from build123d import *

# Parameters (mm, degrees)
WYTNIJ_WYCI_GNI_CIE1_START = -52
WYTNIJ_WYCI_GNI_CIE1_DEPTH = 72
SZKIC3_R                   = 3
WYTNIJ_WYCI_GNI_CIE2_DEPTH = 12
SZYK_KO_OWY1_COUNT         = 6


with BuildPart() as part:
    # Szkic1 → Obrót1 (revolve)
    with BuildSketch(Plane.XY):
        Polygon((0, -4), (0, -9.4775), (1, -10.4775), (6.5225, -10.4775), (8, -9), (10, -9), (10, -11.1), (10.489897949, -11.5), (10, -12.1), (10, -12.5), (19, -12.5), (19, -15.585), (28.915, -15.585), (32, -12.5), (70, -12.5), (70, -11.3155), (68, -9.3155), (54, -9.3155), (53, -10.5), (50, -10.5), (50, -8.5), (19, -8.5), (19, -8.1), (22, -5), (19, -5), (19, -4), align=None)
    revolve(axis=Axis((0, 0, 0), (1, 0, 0)))

    # Szkic2 → Wytnij-wyciągnięcie1 (cut)
    with BuildSketch(Plane.ZY.offset(-19).offset(WYTNIJ_WYCI_GNI_CIE1_START)):
        Polygon((-92.411763114, 13.5), (-7.787311795, 13.5), (7.787311795, 13.5), (92.411763114, 13.5), (92.411763114, 182.748902638), (-92.411763114, 182.748902638), align=None)
    wytnij_wyci_gni_cie1 = extrude(amount=WYTNIJ_WYCI_GNI_CIE1_DEPTH, mode=Mode.SUBTRACT)

    # Szkic3 → Wytnij-wyciągnięcie2 (cut)
    with BuildSketch(Plane(origin=(0, 13.5, 0), x_dir=(1, 0, 0), z_dir=(0, 1, 0))):
        with Locations((25, 0)):
            Circle(SZKIC3_R)
    wytnij_wyci_gni_cie2 = extrude(amount=-WYTNIJ_WYCI_GNI_CIE2_DEPTH, mode=Mode.SUBTRACT)

    # Szyk kołowy1: Wytnij-wyciągnięcie1, Wytnij-wyciągnięcie2 ×6 about axis
    szyk_ko_owy1_axis = Axis((0, 0, 0), (-1, 0, 0))
    for i in range(1, SZYK_KO_OWY1_COUNT):
        add(wytnij_wyci_gni_cie1.rotate(szyk_ko_owy1_axis, i * 360 / SZYK_KO_OWY1_COUNT), mode=Mode.SUBTRACT)
        add(wytnij_wyci_gni_cie2.rotate(szyk_ko_owy1_axis, i * 360 / SZYK_KO_OWY1_COUNT), mode=Mode.SUBTRACT)


solid = part.part
For this review, take the finished solid that the model builds, in its own axes (mm). A direction names the side the tool comes from. Coordinates: 2 decimals unless noted, no trailing zeros. Order: outer loops, then holes, each group sorted by start corner. A loop starts at its lowest first (then second) coordinate and runs counter-clockwise, first axis right, second up. Notation, with made-up numbers: (46.25, -20) -> (55.25, -20) arc R25 ccw to (55.25, 5) -> close; hole circle Ø3 at (-7.5, -39.75). An arc over 180 degrees is marked (long way). Return JSON: item names as keys, results as strings.
1. We need section C-C on x = 52. Write out the cut boundary in (y, z), and give its area (3 significant figures).
Answer block:
{"outline": "circle Ø25 at (0, 0); hole circle Ø21 at (0, 0)", "area": "145 mm²"}
2. For pin 1 Ø3 at (y, z) = (9.5, -12.5) entering from +X; pin 2 Ø6.5 at (y, z) = (-4, -3.5) entering from +X; pin 3 Ø6 at (x, y) = (38.5, 1) entering from -Z; pin 4 Ø4 at (y, z) = (9.5, 9.5) entering from -X, all flat-tipped, find the tip position at first contact; note any pin that passes through.
Answer block:
{"pin 1": "through", "pin 2": "x = 50", "pin 3": "z = -12.5", "pin 4": "x = 10"}
3. We need section B-B on z = 0. State how many separate pieces and enclosed holes the cut face has, and give its area (3 significant figures).
Answer block:
{"separate pieces": "4", "enclosed holes": "0", "area": "610 mm²"}
4. We need section D-D on x = 38. Write out the cut boundary in (y, z).
Answer block:
{"outline": "circle Ø25 at (0, 0); hole circle Ø17 at (0, 0)"}
5. Machinability: for faces 5 (the cylindrical face through (14.563, -11.923, -3.755)), 6 (the cylindrical face through (20.48, 1.08, 4.88)), 7 (the cylindrical face through (24.61, -7.96, -7.84)), which of the approach directions +Z, -Z, +X, -X, +Y, -Y give a long, thin tool a straight path to every point of the face, cutting with its end or side? Answer none if there is none.
Answer block:
{"face 5": "-X", "face 6": "+X", "face 7": "none"}
6. For line 1 (Y direction, x = 57, z = 0); line 2 (Z direction, x = 51.2, y = 0); line 3 (X direction, y = -9.7, z = 0), list the stretches that pass through material, from the lowest coordinate up. Write a range as from..to.
Answer block:
{"line 1": "-12.5..-9.32, 9.32..12.5", "line 2": "-12.5..-10.5, 10.5..12.5", "line 3": "0.22..7.3, 10..22, 28..50, 53.68..68.38"}
7. We need section A-A on x = 20. Write out the cut boundary in (y, z) (3 decimals).
Answer block:
{"outline": "(-13.5, -7.787) arc R15.585 ccw to (-13.494, -7.798) -> (-0.006, -15.585) arc R15.585 ccw to (0.006, -15.585) -> (13.494, -7.798) arc R15.585 ccw to (13.5, -7.787) -> (13.5, 7.787) arc R15.585 ccw to (13.494, 7.798) -> (0.006, 15.585) arc R15.585 ccw to (-0.006, 15.585) -> (-13.494, 7.798) arc R15.585 ccw to (-13.5, 7.787) -> close; circle Ø14.133 at (0, 0); hole circle Ø17 at (0, 0); hole circle Ø10 at (0, 0)"}
8. The part is to be moulded in two halves that separate along X. For faces 1 (the cylindrical face through (9.014, 1.172, -8.923)), 2 (the cylindrical face through (3.8, 1.36, -10.39)), 3 (the cylindrical face through (24.6, 2.8, -10.8)), 4 (the conical face through (21.854, -4.913, -1.547)), say which applies: +X half, -X half, draft (parallel to the pull), parting line (faces both ways), or undercut.
Answer block:
{"face 1": "undercut", "face 2": "draft", "face 3": "undercut", "face 4": "+X half"}
